Could you check a few things on this drawing? It's one solid part, dimensions in mm from its lowest x, y, z. A direction names the side the tool comes from. Coordinates: 2 decimals unless noted, no trailing zeros. Order: outer loops, then holes, each group sorted by start corner. A loop starts at its lowest first (then second) coordinate and runs counter-clockwise, first axis right, second up. Notation, with made-up numbers: (12.25, 30) - (58.25, 30) arc R25 ccw to (58.25, 63) - close; hole circle Ø11 at (21.5, 65.25). An arc over 180 degrees is marked (long way). Answer in a Markdown table with one row per item. Add a question column.
Item 1: Will these pins go through, and if not, where does the flat tip stop? pin 1 Ø24 at (y, z) = (161.5, 47) entering from -X; pin 2 Ø1 at (y, z) = (127, 40.5) entering from +X; pin 3 Ø8.5 at (x, y) = (143.5, 87.5) entering from +Z.
Item 2: On a 3-axis mill with a long thin cutter (end or side, diameter ignored), from which of +Z, -Z, +X, -X, +Y, -Y can I reach the whole of each face in a straight line? I mean the marked faces 1, 2 and 3. Say none if no direction works.
Item 3: I want a section at C-C (z = 19). Please give me the cut outline in (x, y), plus the area to 3 significant figures.
Item 4: If I drill on line 1 along Y through (x, z) = (5, 1); line 2 along X through (y, z) = (187, 1.2); line 3 along X through (y, z) = (142, 40.5), over which ranges is the centre line in solid material (lowest first)? Write a range as from..to.
Item 5: I want a section at B-B (y = 187). Please give me the cut outline in (x, z).
Item 6: I want a section at A-A (x = 141.75). Please give me the cut outline in (y, z), plus the area to 3 significant figures.
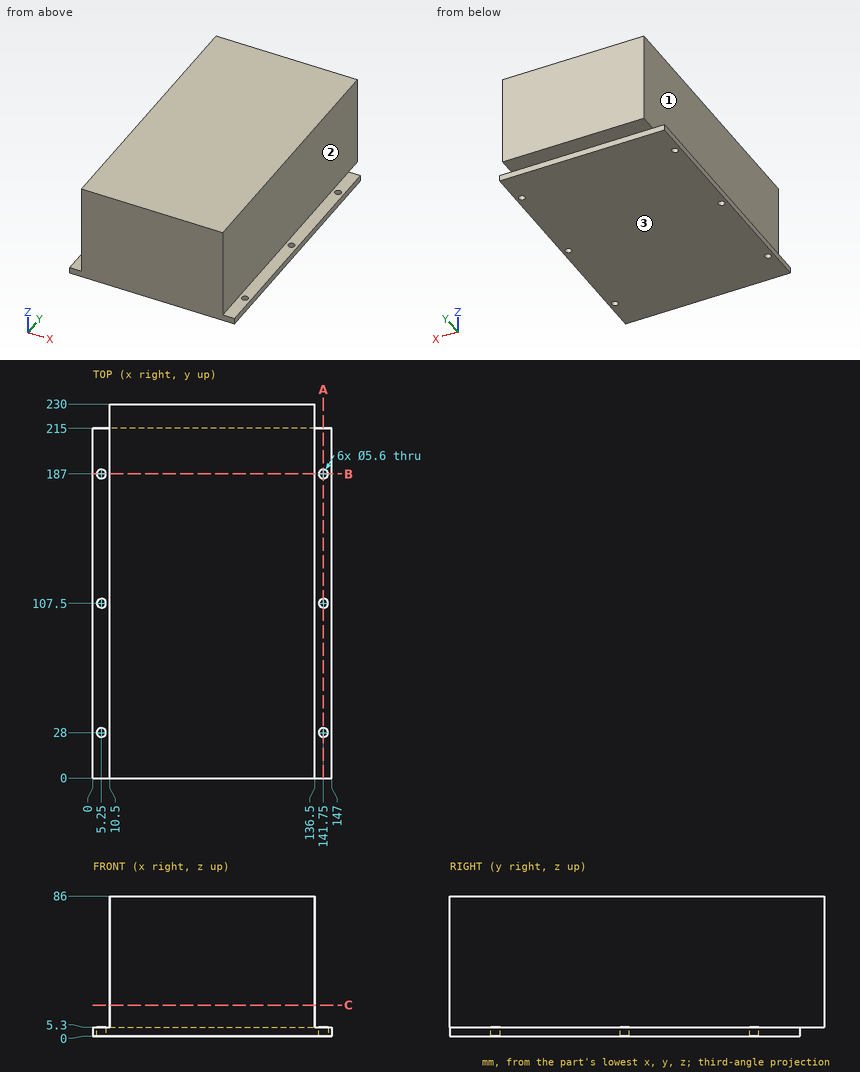
Values follow:
| question | item | result |
|---|---|---|
| 1 | pin 1 | stops at x = 10.5 |
| 1 | pin 2 | stops at x = 136.5 |
| 1 | pin 3 | stops at z = 5.3 |
| 2 | face 1 | +Z, -X, +Y, -Y |
| 2 | face 2 | +Z, +X, +Y, -Y |
| 2 | face 3 | -Z, +X, -X, +Y, -Y |
| 3 | outline | (10.5, 0) - (136.5, 0) - (136.5, 230) - (10.5, 230) - close |
| 3 | area | 29,000 mm^2 |
| 4 | line 1 | y = 0..25.21, 30.79..104.71, 110.29..184.21, 189.79..215 |
| 4 | line 2 | x = 0..2.45, 8.05..138.95, 144.55..147 |
| 4 | line 3 | x = 10.5..136.5 |
| 5 | outline | (0, 0) - (2.45, 0) - (2.45, 5.3) - (0, 5.3) - close; (8.05, 0) - (138.95, 0) - (138.95, 5.3) - (136.5, 5.3) - (136.5, 86) - (10.5, 86) - (10.5, 5.3) - (8.05, 5.3) - close; (144.55, 0) - (147, 0) - (147, 5.3) - (144.55, 5.3) - close |
| 6 | outline | (0, 0) - (25.2, 0) - (25.2, 5.3) - (0, 5.3) - close; (30.8, 0) - (104.7, 0) - (104.7, 5.3) - (30.8, 5.3) - close; (110.3, 0) - (184.2, 0) - (184.2, 5.3) - (110.3, 5.3) - close; (189.8, 0) - (215, 0) - (215, 5.3) - (189.8, 5.3) - close |
| 6 | area | 1,050 mm^2 |
